Geometry: final body of the model. Coordinates: model frame, mm. A direction names the side the tool comes from. Round coordinates to 2 decimals unless told otherwise and drop trailing zeros. Loops run counter-clockwise (first coordinate to the right, second up) from the corner with the lowest first, then second, coordinate; pieces in that order, holes last. Notation, with made-up numbers: M -31,53 L 10,53 A26 cw 10,70 Z; hole C 70.5,-20.75 d9. An arc over 180 degrees is marked long. Write each question's results on one line, items separated by ' | '.
```python
from build123d import *

# Parameters (mm, degrees)
F0_W     = 61
F0_H     = 61
F0_R     = 5
F1_DEPTH = 5
F2_W     = 61
F2_H     = 61
F2_W_2   = 58
F2_H_2   = 58
F3_DEPTH = 25
F4_R     = 2.5
F5_DEPTH = 1.5


with BuildPart() as f1:
    # F0 (on Top) → F1 (new body)
    with BuildSketch(Plane.XY):
        with Locations((22.5, 22.5)):
            Rectangle(F0_W, F0_H)
        Circle(F0_R, mode=Mode.SUBTRACT)
        with Locations((15, 0)):
            Circle(F0_R, mode=Mode.SUBTRACT)
        with Locations((0, 15)):
            Circle(F0_R, mode=Mode.SUBTRACT)
        with Locations((15, 15)):
            Circle(F0_R, mode=Mode.SUBTRACT)
        with Locations((30, 0)):
            Circle(F0_R, mode=Mode.SUBTRACT)
        with Locations((45, 0)):
            Circle(F0_R, mode=Mode.SUBTRACT)
        with Locations((30, 15)):
            Circle(F0_R, mode=Mode.SUBTRACT)
        with Locations((45, 15)):
            Circle(F0_R, mode=Mode.SUBTRACT)
        with Locations((0, 30)):
            Circle(F0_R, mode=Mode.SUBTRACT)
        with Locations((15, 30)):
            Circle(F0_R, mode=Mode.SUBTRACT)
        with Locations((0, 45)):
            Circle(F0_R, mode=Mode.SUBTRACT)
        with Locations((15, 45)):
            Circle(F0_R, mode=Mode.SUBTRACT)
        with Locations((30, 30)):
            Circle(F0_R, mode=Mode.SUBTRACT)
        with Locations((45, 30)):
            Circle(F0_R, mode=Mode.SUBTRACT)
        with Locations((30, 45)):
            Circle(F0_R, mode=Mode.SUBTRACT)
        with Locations((45, 45)):
            Circle(F0_R, mode=Mode.SUBTRACT)
    extrude(amount=F1_DEPTH)

    # F2 (on face) → F3 (join)
    with BuildSketch(Plane.XY.offset(5)):
        with Locations((22.5, 22.5)):
            Rectangle(F2_W, F2_H)
        with Locations((22.5, 22.5)):
            Rectangle(F2_W_2, F2_H_2, mode=Mode.SUBTRACT)
    extrude(amount=F3_DEPTH)

    # F4 (on face) → F5 (cut, through all)
    with BuildSketch(Plane.XZ.offset(8)):
        with Locations((22.101691, 26.540134)):
            Circle(F4_R)
        with Locations((12.705106, 8.884987)):
            Circle(F4_R)
        with Locations((32.693203, 9.574879)):
            Circle(F4_R)
    extrude(amount=-F5_DEPTH, mode=Mode.SUBTRACT)


solid = f1.part
```
1. Section D-D (z = 10.5). Output: boundary loops of the cut face in (x, y), then the cut area to 3 significant figures.
Answer key:
outline: M -8,-8 L 10.8,-8 L 10.8,-6.5 L -6.5,-6.5 L -6.5,51.5 L 51.5,51.5 L 51.5,-6.5 L 35.02,-6.5 L 35.02,-8 L 53,-8 L 53,53 L -8,53 Z; M 14.61,-8 L 30.37,-8 L 30.37,-6.5 L 14.61,-6.5 Z | area: 344 mm²
2. Section A-A (y = 12). Output: boundary loops of the cut face in (x, z), then the cut area to 3 significant figures.
Answer key:
outline: M -8,0 L -4,0 L -4,5 L -6.5,5 L -6.5,30 L -8,30 Z; M 4,0 L 11,0 L 11,5 L 4,5 Z; M 19,0 L 26,0 L 26,5 L 19,5 Z; M 34,0 L 41,0 L 41,5 L 34,5 Z; M 49,0 L 53,0 L 53,30 L 51.5,30 L 51.5,5 L 49,5 Z | area: 220 mm²
3. Section C-C (x = 0). Output: boundary loops of the cut face in (y, z), then the cut area to 3 significant figures.
Answer key:
outline: M -8,0 L -5,0 L -5,5 L -6.5,5 L -6.5,30 L -8,30 Z; M 5,0 L 10,0 L 10,5 L 5,5 Z; M 20,0 L 25,0 L 25,5 L 20,5 Z; M 35,0 L 40,0 L 40,5 L 35,5 Z; M 50,0 L 53,0 L 53,30 L 51.5,30 L 51.5,5 L 50,5 Z | area: 180 mm²
4. Access query for faces 4 (the face through (22, -6.5, 17)), 5 (the face through (10.208, -7.26, 8.995)), 6 (the face through (41, 12, 2)). Directions: +Z, -Z, +X, -X, +Y, -Y. A direction counts if a zero-diameter tool reaches every point of the face in a straight line with its end or side. Return the directions, or none.
Answer key:
face 4: +Z | face 5: -Y | face 6: +Z, -Z
5. Pin query (flat end, axial travel): P1, Ø6, axis at x = 15, y = 30, coming from the -Z side; P2, Ø16, axis at x = 45, y = 45, coming from the +Z side. Return the tip coordinate at first contact, or that it passes through.
Answer key:
P1: passes through | P2: stops at z = 30
6. Draft query along Y for faces 1 (the face through (41, 27, 2)), 2 (the face through (22, 53, 15)), 3 (the face through (-8, 22, 15)). Return one class per face: pulls with the +Y half, pulls with the -Y half, needs draft (parallel to the pull), parting line crosses it, or undercut.
Answer key:
face 1: undercut | face 2: pulls with the +Y half | face 3: needs draft
7. Ray query, probe 1 along Y at (x, z) = (30, 2.1); probe 2 along X at (y, z) = (5.5, 14.75). Return the intervals inside material, ascending.
Answer key:
probe 1: y = -8 to -5, 5 to 10, 20 to 25, 35 to 40, 50 to 53 | probe 2: x = -8 to -6.5, 51.5 to 53
8. Section B-B (z = 17.5). Output: boundary loops of the cut face in (x, y).
Answer key:
outline: M -8,-8 L 53,-8 L 53,53 L -8,53 Z; hole M -6.5,-6.5 L 51.5,-6.5 L 51.5,51.5 L -6.5,51.5 Z
